Build history of the part. All positions in model axes, mm. Give positions to 0.01 mm unless a question says otherwise; leave off trailing zeros. Write each loop counter-clockwise with the first axis right and the second up, starting at its lowest first coordinate (ties: lowest second). Pieces come first, ordered by that corner, then holes. Notation, with made-up numbers: M 76.25,12.25 L 108.25,12.25 A29 cw 108.25,46.25 Z; hole C 19.5,87 d9. An arc over 180 degrees is marked long. Return JSON: item names as keys, results as strings. Group by question number.
Q1. Flat gauge pins, fed straight in: pin 1 Ø2 at (y, z) = (2.5, 2.5) entering from +X; pin 2 Ø3 at (y, z) = (-9.5, 3) entering from +X; pin 3 Ø1.5 at (x, z) = (28.5, 1.5) entering from +Y. Where does each tip first touch, or does it go through?
Q2. Band-saw the part on D-D, the plane x = 25. Give the cut face in (y, z).
Q3. Wall check: probe 1 along Y at (x, z) = (54, 2.25); probe 2 along Y at (x, z) = (52, 3.5); probe 3 along X at (y, z) = (-3.25, 3.5). Give the ranges that are in metal, low to high.
Q4. Band-saw the part on A-A, the plane x = 167. Give the cut face in (y, z), then the cut area to 3 significant figures.
Q5. Band-saw the part on B-B, the plane x = 213. Give the cut face in (y, z), then the cut area to 3 significant figures.
Q6. Band-saw the part on C-C, the plane z = 2.5. Count the separate pieces of the cut face and the enclosed holes in it, then the cut area to 3 significant figures.
from build123d import *

# Parameters (mm, degrees)
CROQUIS1_R              = 13.5
SALIENTE_EXTRUIR1_DEPTH = 6.35
CORTAR_EXTRUIR1_DEPTH   = 6.35
CORTAR_EXTRUIR3_DEPTH   = 10
CROQUIS4_R              = 1.5
CROQUIS4_R_2            = 2
CORTAR_EXTRUIR4_DEPTH   = 10
CROQUIS5_R              = 1.5
CORTAR_EXTRUIR5_DEPTH   = 7.35
CROQUIS6_R              = 1.5
CORTAR_EXTRUIR6_DEPTH   = 7.35


with BuildPart() as part:
    # Croquis1 → Saliente-Extruir1 (new body)
    with BuildSketch(Plane.XY):
        Circle(CROQUIS1_R)
        with BuildLine():
            Line((85, 15), (45, 15))
            Line((45, 15), (-0.447526726, 13.492580177))
            ThreePointArc((-0.447526726, 13.492580177), (9.386383468, 9.702876141), (13.5, 0))
            ThreePointArc((13.5, 0), (9.386383468, -9.702876141), (-0.447526726, -13.492580177))
            Line((-0.447526726, -13.492580177), (45, -15))
            Line((45, -15), (85, -15))
            Line((85, -15), (110, -12.5))
            Line((110, -12.5), (160, -12.5))
            Line((160, -12.5), (185, -15))
            Line((185, -15), (225, -15))
            Line((225, -15), (270.447526726, -13.492580177))
            ThreePointArc((270.447526726, -13.492580177), (256.5, 0), (270.447526726, 13.492580177))
            Line((270.447526726, 13.492580177), (225, 15))
            Line((225, 15), (185, 15))
            Line((185, 15), (160, 12.5))
            Line((160, 12.5), (110, 12.5))
            Line((110, 12.5), (85, 15))
        make_face()
        with Locations((270, 0)):
            Circle(CROQUIS1_R)
    extrude(amount=SALIENTE_EXTRUIR1_DEPTH)

    # Croquis2 → Cortar-Extruir1 (cut)
    with BuildSketch(Plane.XY.offset(6.35)):
        with BuildLine():
            ThreePointArc((5.6, 6.394528911), (0, 8.5), (-5.6, 6.394528911))
            Line((-5.6, 6.394528911), (-5.6, -6.394528911))
            ThreePointArc((-5.6, -6.394528911), (0, -8.5), (5.6, -6.394528911))
            Line((5.6, -6.394528911), (5.6, 6.394528911))
        make_face()
    extrude(amount=-CORTAR_EXTRUIR1_DEPTH, mode=Mode.SUBTRACT)

    # Croquis3 → Cortar-Extruir3 (cut)
    with BuildSketch(Plane.XY.offset(6.35)):
        with BuildLine():
            Line((122.5, 7), (42, 7))
            ThreePointArc((42, 7), (35, 0), (42, -7))
            Line((42, -7), (122.5, -7))
            ThreePointArc((122.5, -7), (129.5, 0), (122.5, 7))
        make_face()
        with BuildLine():
            Line((228, 7), (147.5, 7))
            ThreePointArc((147.5, 7), (140.5, 0), (147.5, -7))
            Line((147.5, -7), (228, -7))
            ThreePointArc((228, -7), (235, 0), (228, 7))
        make_face()
    extrude(amount=-CORTAR_EXTRUIR3_DEPTH, mode=Mode.SUBTRACT)

    # Croquis4 → Cortar-Extruir4 (cut)
    with BuildSketch(Plane.XY.offset(6.35)):
        with Locations((52, 11)):
            Circle(CROQUIS4_R)
        with Locations((52, -11)):
            Circle(CROQUIS4_R)
        with Locations((218, -11)):
            Circle(CROQUIS4_R)
        with Locations((218, 11)):
            Circle(CROQUIS4_R)
        with Locations((135, 0)):
            Circle(CROQUIS4_R_2)
    extrude(amount=-CORTAR_EXTRUIR4_DEPTH, mode=Mode.SUBTRACT)

    # Croquis5 → Cortar-Extruir5 (cut, through all)
    with BuildSketch(Plane.XY.offset(6.35)):
        with Locations((248, 0)):
            Circle(CROQUIS5_R)
    extrude(amount=-CORTAR_EXTRUIR5_DEPTH, mode=Mode.SUBTRACT)

    # Croquis6 → Cortar-Extruir6 (cut, through all)
    with BuildSketch(Plane.XY.offset(6.35)):
        with Locations((250.397856468, 9.987790994)):
            Circle(CROQUIS6_R)
        with Locations((258.509333353, 9.641814145)):
            Circle(CROQUIS6_R)
        with Locations((258.509333353, -9.641814145)):
            Circle(CROQUIS6_R)
        with Locations((250.397856468, -9.987790994)):
            Circle(CROQUIS6_R)
    extrude(amount=-CORTAR_EXTRUIR6_DEPTH, mode=Mode.SUBTRACT)


solid = part.part
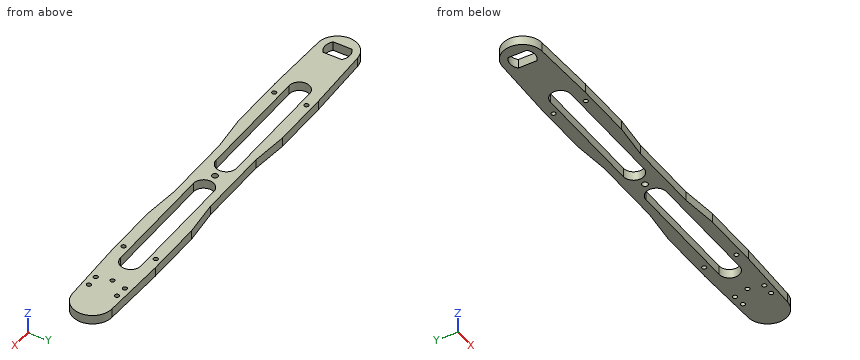
From the geometry:
{
 "1": {"pin 1": "stops at x = 283.42", "pin 2": "stops at x = 280.87", "pin 3": "stops at y = 14.48"},
 "2": {"outline": "M -14.34,0 L 14.34,0 L 14.34,6.35 L -14.34,6.35 Z"},
 "3": {"probe 1": "y = -15 to -7, 7 to 15", "probe 2": "y = -15 to -12.5, -9.5 to -7, 7 to 9.5, 12.5 to 15", "probe 3": "x = -13.1 to -5.6, 5.6 to 35.8, 128.7 to 141.3, 234.2 to 283.1"},
 "4": {"outline": "M -13.2,0 L -7,0 L -7,6.35 L -13.2,6.35 Z; M 7,0 L 13.2,0 L 13.2,6.35 L 7,6.35 Z", "area": "78.7 mm^2"},
 "5": {"outline": "M -15,0 L -7,0 L -7,6.35 L -15,6.35 Z; M 7,0 L 15,0 L 15,6.35 L 7,6.35 Z", "area": "102 mm^2"},
 "6": {"separate pieces": "1", "enclosed holes": "13", "area": "5,350 mm^2"}
}
